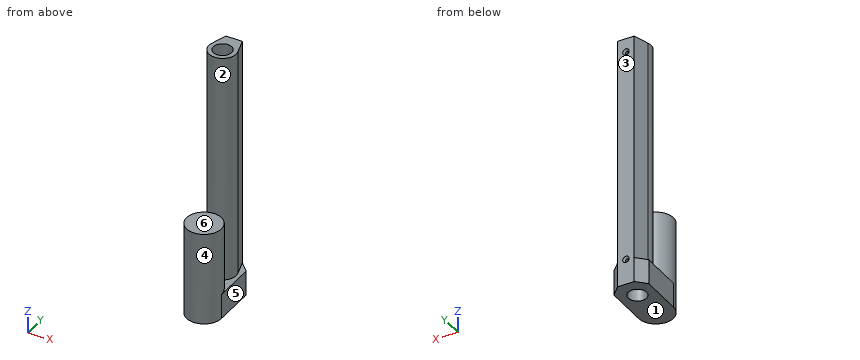
Autodesk Inventor part; units mm, degrees
ref_plane "YZ Plane" through (0, 0, 0) normal (1, 0, 0) x (0, 1, 0)
ref_plane "XZ Plane" through (0, 0, 0) normal (0, 1, 0) x (-1, 0, 0)
ref_plane "XY Plane" through (0, 0, 0) normal (0, 0, 1) x (1, 0, 0)
sketch "Sketch1" plane through (0, 0, 0) normal (0, 0, 1) x (1, 0, 0)
  circle A0 centre (0, 0) radius 14.8
  line L0 (-9, 21.5) -> (9, 21.5)
  line L1 (-9, 21.5) -> (-19, 11.5)
  line L2 (-19, 11.5) -> (-19, -34.776357)
  circle A1 centre (0, -34.5) radius 19
  line L3 (0, 21.5) -> (0, -34.5) construction
  line L4 (9, 21.5) -> (19, 11.5)
  line L5 (19, 11.5) -> (19, -34.776357)
  point P0 (-19, -34.5)
  point P1 (19, -34.5)
  dimension "d0" = 29.6
  dimension "d1" = 18
  dimension "d2" = 21.5
  dimension "d3" = 38
  dimension "d4" = 56
  dimension "d5" = 45
sketch "Sketch1 outline for Extrusion1" plane through (0, 0, 0) normal (0, 0, 1) x (1, 0, 0)
  line L0 (19, 11.5) -> (9, 21.5)
  line L1 (19, -34.5) -> (19, 11.5)
  arc A0 (-19, -34.5) -> (19, -34.5) centre (0, -34.5) ccw
  line L2 (-19, 11.5) -> (-19, -34.5)
  line L3 (-9, 21.5) -> (-19, 11.5)
  line L4 (9, 21.5) -> (-9, 21.5)
extrude "Extrusion1" add sketch "Sketch1 outline for Extrusion1" along normal blind 27
sketch "Sketch2" plane through (0, 0, 27) normal (0, 0, 1) x (1, 0, 0)
  line L0 (9, 21.5) -> (-9, 21.5)
  circle A0 centre (0, 0) radius 14.8
  line L1 (-9, 21.5) -> (-14.175455, 4.253996)
  line L2 (9, 21.5) -> (14.175455, 4.253996)
  line L3 (9, 21.5) -> (-9, 21.5)
  line L4 (-9, 21.5) -> (9, 21.5)
  dimension "d8" = 29.6
extrude "Extrusion2" add sketch "Sketch2" along normal blind 250
sketch "Sketch3" plane through (0, 0, 27) normal (0, 0, 1) x (1, 0, 0)
  arc A0 (-19, -34.5) -> (19, -34.5) centre (0, -34.5) ccw
  circle A1 centre (0, -34.5) radius 19
  point P0 (0, 0)
  point P1 (19, -34.5)
  point P2 (-19, -34.5)
extrude "Extrusion3" add sketch "Sketch3" along normal blind 74
sketch "Sketch4" plane through (-9, 21.5, 0) normal (0, 1, 0) x (1, 0, 0)
  line L0 (18, 0) -> (0, 0)
  line L1 (0, 0) -> (0, -27)
  line L2 (0, -27) -> (0, -277)
  line L3 (18, -277) -> (0, -277)
  line L4 (18, -27) -> (18, -277)
  line L5 (18, 0) -> (18, -27)
  line L6 (-16, -266.5) -> (34, -266.5)
  point P0 (9, 0)
  point P1 (9, -266.5)
  point P2 (9, -277)
  dimension "d13" = 50
  dimension "d14" = 10.5
split_face "Split1"
sketch "Sketch5" plane through (0, 0, 277) normal (0, 0, 1) x (1, 0, 0)
  circle A0 centre (0, 0) radius 10
  dimension "d15" = 20
extrude "Extrusion4" cut sketch "Sketch5" against normal blind 427
sketch "Sketch6" plane through (-9, 21.5, 0) normal (0, 1, 0) x (1, 0, 0)
  line L0 (18, -266.5) -> (0, -266.5)
  line L1 (18, -27) -> (18, -266.5)
  line L2 (18, 0) -> (18, -27)
  line L3 (18, 0) -> (0, 0)
  line L4 (0, 0) -> (0, -27)
  line L5 (0, -27) -> (0, -266.5)
  line L6 (18, -266.5) -> (0, -266.5)
  line L7 (0, -266.5) -> (0, -277)
  line L8 (18, -277) -> (0, -277)
  line L9 (18, -266.5) -> (18, -277)
  point P0 (9, 0)
  point P1 (9, -262)
  point P2 (9, -28)
  point P3 (9, 0)
  point P4 (9, -277)
  dimension "d18" = 28
  dimension "d19" = 15
hole "Hole1" at (0, 21.5, 262) at (0, 21.5, 28) direction (0, -1, 0) diameter 3.242 depth 8 countersink diameter 7 countersink angle 90
properties part number "Linear Motor (T-Frame)" material "Aluminum 6061"
Can you work these out from the model? Positions are in its coordinate system, mm. Face numbers are marked on the shaded views. A direction names the side the tool comes from. Round coordinates to 2 decimals unless told otherwise and drop trailing zeros. Order: outer loops, then holes, each group sorted by start corner. A loop starts at its lowest first (then second) coordinate and runs counter-clockwise, first axis right, second up.
(1) If we section it at C-C (y = -40): Please give me the cut outline in (x, z).
Results are:
outline: (-18.19, 0) - (18.19, 0) - (18.19, 101) - (-18.19, 101) - close
(2) If I drill on L1, parallel to Z at x = 0, y = 15.75; L2, parallel to Y at x = 0, z = 142; L3, parallel to Y at x = 8, z = 66.5, over which ranges is the centre line in solid material (lowest first)?
Results are:
L1: z = 0 to 26.38, 29.62 to 260.38, 263.62 to 277
L2: y = -14.8 to -10, 10 to 21.5
L3: y = -51.73 to -17.27, -12.45 to -6, 6 to 21.5
(3) If we section it at B-B (y = 0): Please give me the cut outline in (x, z).
Results are:
outline: (-19, 0) - (-10, 0) - (-10, 277) - (-14.8, 277) - (-14.8, 27) - (-19, 27) - close; (10, 0) - (19, 0) - (19, 27) - (14.8, 27) - (14.8, 277) - (10, 277) - close
(4) If we section it at A-A (z = 85.5): Please give me the cut outline in (x, y).
Results are:
outline: circle Ø38 at (0, -34.5); (-14.18, 4.25) arc R14.8 ccw (long way) to (14.18, 4.25) - (9, 21.5) - (-9, 21.5) - close; hole circle Ø20 at (0, 0)
(5) I'm going to push flat-ended pins straight in: pin 1 (1.5 mm diameter, centred on x = -0.5, y = -31, fed in from +Z); pin 2 (5 mm diameter, centred on x = 0, z = 28, fed in from -Y); pin 3 (2 mm diameter, centred on x = 11.5, z = 109, fed in from -Y); pin 4 (6 mm diameter, centred on y = -25, z = 105.5, fed in from +X). Where does each tip first touch, or does it pass through?
Results are:
pin 1: stops at z = 101
pin 2: stops at y = -53.5
pin 3: stops at y = -10.43
pin 4: passes through
(6) We'd pull the mould along Y, two halves only. Please class the marked faces 1, 2 and 3: +Y half, -Y half, draft (parallel to the pull), parting line (faces both ways), or undercut.
Results are:
face 1: draft
face 2: undercut
face 3: +Y half
(7) On a 3-axis mill with a long thin cutter (end or side, diameter ignored), from which of +Z, -Z, +X, -X, +Y, -Y can I reach the whole of each face in a straight line? I mean the marked faces 4, 5 and 6. Say none if no direction works.
Results are:
face 4: +Z
face 5: +Z, -Z, +X, +Y, -Y
face 6: +Z, +X, -X, -Y
